For this review, take the finished solid that the model builds, in its own axes (mm). Face numbers are marked on the shaded views. A direction names the side the tool comes from. Coordinates: 2 decimals unless noted, no trailing zeros. Write each loop counter-clockwise with the first axis right and the second up, starting at its lowest first coordinate (ties: lowest second). Pieces come first, ordered by that corner, then holes. Notation, with made-up numbers: (13, -32.5) -> (57, -32.5) arc R18 ccw to (57, 2.5) -> close; hole circle Ø3 at (-30, 21.5). An arc over 180 degrees is marked (long way). One line per item, written item: value. Start each with the question number.
1) For pin 1 Ø2 at (y, z) = (-18.5, 5.5) entering from -X; pin 2 Ø12 at (x, y) = (-11.5, -15) entering from +Z; pin 3 Ø0.8 at (x, z) = (-17.5, 6.5) entering from +Y, all flat-tipped, find the tip position at first contact; note any pin that passes through.
2) Add section A-A (x = -1.5). State the section outline as (y, z) points.
3) For probe 1 along Y at (x, z) = (1, 8); probe 2 along X at (y, z) = (10.5, 1.75); probe 3 along X at (y, z) = (0.5, 1.5), list the stretches that pass through material, from the lowest coordinate up. Write a range as from..to.
4) Mouldability with a two-part tool opening along Y and no side actions: class the marked faces 1, 2 and 3 as released by +Y, released by -Y, zero draft, split by the parting line, or undercut.
5) Add section C-C (y = -22). State the section outline as (x, z) points.
6) Add section B-B (y = -13). State the section outline as (x, z) points.
7) Machinability: for the marked faces 4, 5 and 6, which of the approach directions +Z, -Z, +X, -X, +Y, -Y give a long, thin tool a straight path to every point of the face, cutting with its end or side? Answer none if there is none.
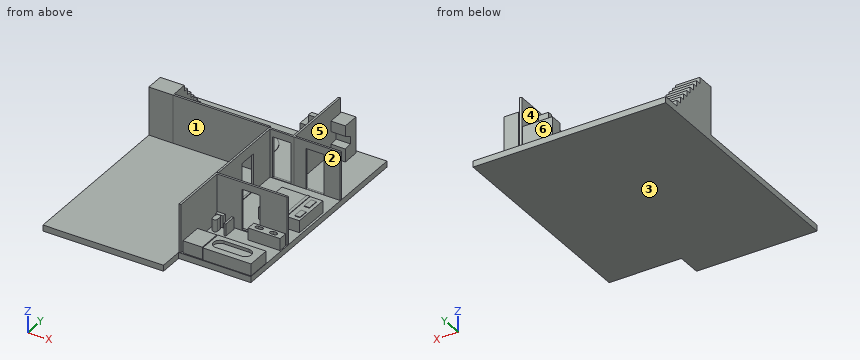
from build123d import *

# Parameters (mm, degrees)
PAD_DEPTH       = 1
PAD004_DEPTH    = 8
PAD005_DEPTH    = 4
SKETCH014_W     = 7.729191
SKETCH014_H     = 0.31886
PAD006_DEPTH    = 8
SKETCH015_W     = 11.953097
SKETCH015_H     = 0.33
PAD007_DEPTH    = 8
SKETCH016_W     = 3
SKETCH016_H     = 6.672529
POCKET_DEPTH    = 5
SKETCH017_W     = 3.102198
SKETCH017_H     = 6.756484
POCKET001_DEPTH = 5
SKETCH018_W     = 15.99927
SKETCH018_H     = 0.33
PAD008_DEPTH    = 8
SKETCH020_W     = 3
SKETCH020_H     = 6.100988
POCKET002_DEPTH = 5
PAD009_DEPTH    = 8
SKETCH005_W     = 5.295486
SKETCH005_H     = 1.5
SKETCH005_W_2   = 8
SKETCH005_H_2   = 4
SKETCH005_W_3   = 3.212604
SKETCH005_H_3   = 3.838312
SKETCH005_W_4   = 1.267163
SKETCH005_H_4   = 0.540659
SKETCH005_W_5   = 0.33
SKETCH005_H_5   = 2.119946
PAD010_DEPTH    = 2
POCKET003_DEPTH = 0.5
SKETCH024_W     = 6.8
SKETCH024_H     = 6.2
PAD011_DEPTH    = 2
SKETCH025_W     = 2.4
SKETCH025_H     = 2.8
PAD012_DEPTH    = 6
POCKET004_DEPTH = 2.5
SKETCH028_W     = 3
SKETCH028_H     = 6.730199
POCKET005_DEPTH = 5
PAD013_DEPTH    = 3.2
POCKET006_DEPTH = 0.5
SKETCH031_W     = 1.637633
SKETCH031_H     = 0.834874
PAD014_DEPTH    = 1.2
PAD015_DEPTH    = 0.1
SKETCH033_W     = 0.866982
SKETCH033_H     = 1.862408
SKETCH033_W_2   = 0.866983
SKETCH033_H_2   = 1.637636
SKETCH033_W_3   = 0.481657
SKETCH033_H_3   = 6.036772
PAD016_DEPTH    = 0.1


with BuildPart() as part:
    # Sketch → Pad (new body)
    with BuildSketch(Plane.XY):
        Polygon((0, -28), (-20, -28), (-20, 0), (-16, 0), (-16, 12), (12, 12), (12, -24), (0, -24), align=None)
    extrude(amount=PAD_DEPTH)

    # Sketch007 → Pad004 (join)
    with BuildSketch(Plane.XY.offset(1)):
        Polygon((0.316723, -0.33), (0.316723, -13.888312), (0, -13.888312), (0, 0), (4, 0), (4, 11.732385), (4.33, 11.969152), (4.33, -0.33), align=None)
    extrude(amount=PAD004_DEPTH)

    # Sketch004 (on Face4 of Pad) → Pad005 (join)
    with BuildSketch(Plane(origin=(-16, 0, 0), x_dir=(0, -1, 0), z_dir=(-1, 0, 0))):
        Polygon((-12, 0), (-12, 1), (-9, 1), (-9, 2), (-8.142857, 2), (-8.142857, 3), (-7.285714, 3), (-7.285714, 4), (-6.428571, 4), (-6.428571, 5), (-5.571429, 5), (-5.571429, 6), (-4.714286, 6), (-4.714286, 7), (-3.857143, 7), (-3.857143, 8), (-3, 8), (-3, 9), (0, 9), (0, 0), align=None)
    extrude(amount=PAD005_DEPTH)

    # Sketch014 (on Face5 of Pad005) → Pad006 (join)
    with BuildSketch(Plane.XY.offset(1)):
        with Locations((8.106394, -0.15943)):
            Rectangle(SKETCH014_W, SKETCH014_H)
    extrude(amount=PAD006_DEPTH)

    # Sketch015 (on Face5 of Pad006) → Pad007 (join)
    with BuildSketch(Plane.XY.offset(1)):
        with Locations((5.976548, -14.165)):
            Rectangle(SKETCH015_W, SKETCH015_H)
    extrude(amount=PAD007_DEPTH)

    # Sketch016 (on Face16 of Pad007) → Pocket (cut)
    with BuildSketch(Plane.XZ.offset(14.33)):
        with Locations((5.939301, 4.490863)):
            Rectangle(SKETCH016_W, SKETCH016_H)
    extrude(amount=-POCKET_DEPTH, mode=Mode.SUBTRACT)

    # Sketch017 (on Face19 of Pocket) → Pocket001 (cut)
    with BuildSketch(Plane.XZ.offset(0.33)):
        with Locations((2.28487, 4.481079)):
            Rectangle(SKETCH017_W, SKETCH017_H)
    extrude(amount=-POCKET001_DEPTH, mode=Mode.SUBTRACT)

    # Sketch018 (on Face5 of Pocket001) → Pad008 (join)
    with BuildSketch(Plane.XY.offset(1)):
        with Locations((-7.999635, 0.165)):
            Rectangle(SKETCH018_W, SKETCH018_H)
    extrude(amount=PAD008_DEPTH)

    # Sketch020 (on Face20 of Pad008) → Pocket002 (cut)
    with BuildSketch(Plane(origin=(0, 0, 0), x_dir=(0, -1, 0), z_dir=(-1, 0, 0))):
        with Locations((6.176963, 4.163983)):
            Rectangle(SKETCH020_W, SKETCH020_H)
    extrude(amount=-POCKET002_DEPTH, mode=Mode.SUBTRACT)

    # Sketch021 (on Face5 of Pocket002) → Pad009 (join)
    with BuildSketch(Plane.XY.offset(1)):
        Polygon((0, -14.263546), (0, -23.894106), (0.33, -23.872581), (0.33, -14.263546), align=None)
    extrude(amount=PAD009_DEPTH)

    # Sketch005 (on Face5 of Pad009) → Pad010 (join)
    with BuildSketch(Plane.XY.offset(1)):
        with Locations((9.181875, -15.260856)):
            Rectangle(SKETCH005_W, SKETCH005_H)
        with Locations((7.922637, -21.844449)):
            Rectangle(SKETCH005_W_2, SKETCH005_H_2)
        with Locations((2.172653, -21.834947)):
            Rectangle(SKETCH005_W_3, SKETCH005_H_3)
        with BuildLine():
            ThreePointArc((1.67577, -15.683133), (1.255132, -15.262495), (0.834494, -15.683133))
            Line((0.834494, -15.683133), (0.834494, -16.314087))
            ThreePointArc((0.834494, -16.314087), (1.255132, -16.734725), (1.67577, -16.314087))
            Line((1.67577, -15.683133), (1.67577, -16.314087))
        make_face()
        with Locations((1.25517, -14.930792)):
            Rectangle(SKETCH005_W_4, SKETCH005_H_4)
        with Locations((3.165, -15.762285)):
            Rectangle(SKETCH005_W_5, SKETCH005_H_5)
    extrude(amount=PAD010_DEPTH)

    # Sketch010 (on Face79 of Pad010) → Pocket003 (cut)
    with BuildSketch(Plane.XY.offset(3)):
        with BuildLine():
            ThreePointArc((5.452506, -20.709412), (4.400786, -21.761133), (5.452506, -22.812854))
            Line((5.452506, -22.812854), (9.654259, -22.812854))
            ThreePointArc((9.654259, -22.812854), (10.70598, -21.761133), (9.654259, -20.709412))
            Line((5.452506, -20.709412), (9.654259, -20.709412))
        make_face()
        with BuildLine():
            ThreePointArc((7.507576, -14.85322), (7.199253, -15.161543), (7.507576, -15.469866))
            Line((7.507576, -15.469866), (8.173935, -15.469866))
            ThreePointArc((8.173935, -15.469866), (8.482258, -15.161543), (8.173935, -14.85322))
            Line((7.507576, -14.85322), (8.173935, -14.85322))
        make_face()
        with BuildLine():
            ThreePointArc((10.044301, -14.90339), (9.689296, -15.258395), (10.044301, -15.6134))
            Line((10.044301, -15.6134), (10.55301, -15.6134))
            ThreePointArc((10.55301, -15.6134), (10.908015, -15.258395), (10.55301, -14.90339))
            Line((10.044301, -14.90339), (10.55301, -14.90339))
        make_face()
    extrude(amount=-POCKET003_DEPTH, mode=Mode.SUBTRACT)

    # Sketch024 (on Face5 of Pocket003) → Pad011 (join)
    with BuildSketch(Plane.XY.offset(1)):
        with Locations((8.22879, -7.462824)):
            Rectangle(SKETCH024_W, SKETCH024_H)
    extrude(amount=PAD011_DEPTH)

    # Sketch025 (on Face5 of Pad011) → Pad012 (join)
    with BuildSketch(Plane.XY.offset(1)):
        with Locations((5.972474, 10.079884)):
            Rectangle(SKETCH025_W, SKETCH025_H)
    extrude(amount=PAD012_DEPTH)

    # Sketch026 (on Face63 of Pad012) → Pocket004 (cut)
    with BuildSketch(Plane.YZ.offset(7.172474)):
        Polygon((8.224654, 3.127523), (10.022843, 3.288076), (9.990732, 4.572494), (8.51365, 5.343146), align=None)
    extrude(amount=-POCKET004_DEPTH, mode=Mode.SUBTRACT)

    # Sketch028 (on Face59 of Pocket004) → Pocket005 (cut)
    with BuildSketch(Plane.XZ.offset(0.31886)):
        with Locations((7.757963, 4.395962)):
            Rectangle(SKETCH028_W, SKETCH028_H)
    extrude(amount=-POCKET005_DEPTH, mode=Mode.SUBTRACT)

    # Sketch029 (on Face5 of Pocket005) → Pad013 (join)
    with BuildSketch(Plane.XY.offset(1)):
        Polygon((-0.991208, 11.715413), (-0.991208, 9.715413), (2.008792, 9.715413), (2.008792, 5.715413), (4.008792, 5.715413), (4.008792, 11.715413), align=None)
    extrude(amount=PAD013_DEPTH)

    # Sketch030 (on Face115 of Pad013) → Pocket006 (cut)
    with BuildSketch(Plane.XY.offset(4.2)):
        with BuildLine():
            ThreePointArc((3.550535, 8.01575), (3.077208, 8.489077), (2.603881, 8.01575))
            Line((2.603881, 8.01575), (2.603881, 7.267244))
            ThreePointArc((2.603881, 7.267244), (3.077208, 6.793917), (3.550535, 7.267244))
            Line((3.550535, 8.01575), (3.550535, 7.267244))
        make_face()
    extrude(amount=-POCKET006_DEPTH, mode=Mode.SUBTRACT)

    # Sketch031 (on Face115 of Pocket006) → Pad014 (join)
    with BuildSketch(Plane.XY.offset(4.2)):
        with Locations((0.690656, 10.93792)):
            Rectangle(SKETCH031_W, SKETCH031_H)
    extrude(amount=PAD014_DEPTH)

    # Sketch032 (on Face5 of Pad014) → Pad015 (join)
    with BuildSketch(Plane.XY.offset(1)):
        with BuildLine():
            ThreePointArc((-9.997042, 9.217286), (-13.309208, 5.90512), (-9.997042, 2.592954))
            Line((-9.997042, 2.592954), (-6.021085, 2.592954))
            ThreePointArc((-6.021085, 2.592954), (-2.708919, 5.90512), (-6.021085, 9.217286))
            Line((-9.997042, 9.217286), (-6.021085, 9.217286))
        make_face()
    extrude(amount=PAD015_DEPTH)

    # Sketch033 (on Face109 of Pad015) → Pad016 (join)
    with BuildSketch(Plane.XY.offset(3)):
        with Locations((10.620443, -6.083477)):
            Rectangle(SKETCH033_W, SKETCH033_H)
        with Locations((10.845216, -9.021587)):
            Rectangle(SKETCH033_W_2, SKETCH033_H_2)
        with Locations((9.271801, -7.432117)):
            Rectangle(SKETCH033_W_3, SKETCH033_H_3)
    extrude(amount=PAD016_DEPTH)


solid = part.part
Numbers:
1. pin 1: x = 0
1. pin 2: z = 1
1. pin 3: y = 4.71
2. outline: (-28, 0) -> (12, 0) -> (12, 1) -> (0.33, 1) -> (0.33, 9) -> (0, 9) -> (0, 1) -> (-28, 1) -> close
3. probe 1: -14.33..-14, -0.33..0
3. probe 2: -0.99..4.33, 4.77..7.17
3. probe 3: -20..-16, 4..4.33
4. face 1: released by -Y
4. face 2: undercut
4. face 3: zero draft
5. outline: (-20, 0) -> (12, 0) -> (12, 1) -> (11.92, 1) -> (11.92, 3) -> (10.68, 3) -> (10.68, 2.5) -> (4.43, 2.5) -> (4.43, 3) -> (3.92, 3) -> (3.92, 1) -> (3.78, 1) -> (3.78, 3) -> (0.57, 3) -> (0.57, 1) -> (0.33, 1) -> (0.33, 9) -> (0, 9) -> (0, 1) -> (-20, 1) -> close
6. outline: (-20, 0) -> (12, 0) -> (12, 1) -> (0.32, 1) -> (0.32, 9) -> (0, 9) -> (0, 1) -> (-20, 1) -> close
7. face 4: +Z
7. face 5: +Z, +Y
7. face 6: +Z, -X, +Y
